Here's how the part is built. I have some questions about the finished solid (model axes, mm). A direction names the side the tool comes from. Coordinates: 2 decimals unless noted, no trailing zeros. Order: outer loops, then holes, each group sorted by start corner. A loop starts at its lowest first (then second) coordinate and runs counter-clockwise, first axis right, second up. Notation, with made-up numbers: M 83.5,-19 L 100.5,-19 A12 ccw 100.5,-14 Z; hole C 77,-19.5 d3. An arc over 180 degrees is marked long. One line per question, with ' | ' between items. Start each with the question number.
```python
from build123d import *

# Parameters (mm, degrees)
BOSS_EXTRUDE1_DEPTH = 3


with BuildPart() as part:
    # Sketch1 → Boss-Extrude1 (new body)
    with BuildSketch(Plane(origin=(0, 0, 0), x_dir=(1, 0, 0), z_dir=(0, 1, 0))):
        with BuildLine():
            Line((-27.566533023, 9.36), (-27.566533023, 0))
            Line((-27.566533023, 0), (-19.823403694, 0))
            ThreePointArc((-19.823403694, 0), (24.20597109, 6.306968985), (65.433466977, 23))
            ThreePointArc((65.433466977, 23), (73.082886665, 22.390495512), (80.646880945, 23.683208869))
            ThreePointArc((80.646880945, 23.683208869), (81.946672363, 24.893615616), (81.784737476, 26.662321164))
            ThreePointArc((81.784737476, 26.662321164), (78.82438559, 31.885442154), (76.202135766, 37.28622747))
            ThreePointArc((76.202135766, 37.28622747), (86.37958616, 41.621825), (95.668579031, 47.629529544))
            ThreePointArc((95.668579031, 47.629529544), (96.113926531, 48.706505439), (95.666017221, 49.782418412))
            ThreePointArc((95.666017221, 49.782418412), (89.924608564, 54.937742393), (85.709789242, 61.401211803))
            ThreePointArc((85.709789242, 61.401211803), (96.000732533, 71.797200989), (102.357305132, 84.971952969))
            ThreePointArc((102.357305132, 84.971952969), (102.11128314, 86.223857216), (101.047487459, 86.928222044))
            ThreePointArc((101.047487459, 86.928222044), (95.950995205, 87.647987285), (90.808707622, 87.869738741))
            ThreePointArc((90.808707622, 87.869738741), (100.106213422, 97.05037675), (104.313081391, 109.420905852))
            ThreePointArc((104.313081391, 109.420905852), (104.396564886, 110.399625231), (103.439203659, 110.619444698))
            ThreePointArc((103.439203659, 110.619444698), (98.285170112, 109.227963636), (93.040390076, 110.224238556))
            ThreePointArc((93.040390076, 110.224238556), (96.824995658, 122.538102913), (96.530215503, 135.417062479))
            ThreePointArc((96.530215503, 135.417062479), (95.551508519, 136.778926007), (93.878347384, 136.893256429))
            ThreePointArc((93.878347384, 136.893256429), (83.613278323, 129.68205398), (77.858466896, 118.535071023))
            ThreePointArc((77.858466896, 118.535071023), (74.985694546, 124.095226744), (72.596248771, 129.879576449))
            ThreePointArc((72.596248771, 129.879576449), (70.378357546, 131.020039942), (68.639848531, 129.231944623))
            ThreePointArc((68.639848531, 129.231944623), (67.651272843, 114.747827583), (68.577278714, 100.25957574))
            ThreePointArc((68.577278714, 100.25957574), (63.407288288, 102.259220756), (59.026108144, 105.655195101))
            ThreePointArc((59.026108144, 105.655195101), (56.300849607, 106.738729111), (54.315586254, 104.580069929))
            ThreePointArc((54.315586254, 104.580069929), (55.34526323, 85.900059583), (63.427341461, 69.02750694))
            Line((63.427341461, 69.02750694), (44.822180162, 73.063888147))
            ThreePointArc((44.822180162, 73.063888147), (43.189327409, 72.023710618), (42.770208924, 70.133600278))
            Line((42.770208924, 70.133600278), (51.693414268, 52.061516653))
            ThreePointArc((51.693414268, 52.061516653), (51.807398335, 49.244580753), (49.792960169, 47.272232126))
            ThreePointArc((49.792960169, 47.272232126), (43.886083409, 53.379891607), (36.716738418, 57.940065925))
            ThreePointArc((36.716738418, 57.940065925), (34.842559279, 58.150522241), (35.17981611, 56.294963797))
            ThreePointArc((35.17981611, 56.294963797), (38.195000716, 47.026649531), (37.963262453, 37.282970301))
            ThreePointArc((37.963262453, 37.282970301), (36.915972263, 35.842205611), (35.471592941, 36.884504997))
            ThreePointArc((35.471592941, 36.884504997), (32.374331301, 43.249850807), (27.655103234, 48.526169922))
            ThreePointArc((27.655103234, 48.526169922), (26.369610718, 48.570167749), (26.028819046, 47.329890419))
            ThreePointArc((26.028819046, 47.329890419), (26.962894841, 38.326203111), (22.69935772, 30.341146196))
            ThreePointArc((22.69935772, 30.341146196), (21.519458622, 30.046407872), (20.701006485, 30.9459459))
            ThreePointArc((20.701006485, 30.9459459), (18.760748853, 37.885894085), (15.830732782, 44.469395153))
            ThreePointArc((15.830732782, 44.469395153), (14.897444009, 44.903650637), (14.219241967, 44.129281378))
            ThreePointArc((14.219241967, 44.129281378), (11.765539078, 35.905199886), (6.117654668, 29.443189676))
            ThreePointArc((6.117654668, 29.443189676), (4.728143423, 29.340639166), (4.041804517, 30.553155976))
            ThreePointArc((4.041804517, 30.553155976), (3.570156048, 36.827406443), (1.56510947, 42.791336307))
            ThreePointArc((1.56510947, 42.791336307), (0.867859685, 43.215318025), (0.196498979, 42.751429503))
            ThreePointArc((0.196498979, 42.751429503), (-10.860043289, 29.237113049), (-27.566533023, 24.16))
            Line((-27.566533023, 24.16), (-27.566533023, 12.36))
            Line((-27.566533023, 12.36), (-16.746533023, 12.36))
            ThreePointArc((-16.746533023, 12.36), (-15.246533023, 10.86), (-16.746533023, 9.36))
            Line((-16.746533023, 9.36), (-27.566533023, 9.36))
        make_face()
    extrude(amount=BOSS_EXTRUDE1_DEPTH)


solid = part.part
```
1. We'd pull the mould along X, two halves only. Please class faces 1 (the face through (-27.567, 1, -5)), 2 (the face through (95.88, 1.48, -71.63)), 3 (the face through (38.175, 1.479, -47.162)), 4 (the face through (47.17, 1.48, -61.22)): released by +X, released by -X, zero draft, split by the parting line, or undercut.
2. Will these pins go through, and if not, where does the flat tip stop? pin 1 (0.9 mm diameter, centred on x = -25, y = 2, fed in from -Z); pin 2 (1 mm diameter, centred on x = 77.5, y = 2, fed in from -Z).
3. Which directions (+Z, -Z, +X, -X, +Y, -Y) give clear straight access to the entire face, cutting with the end or side of a thin tool? Please do faces 5 (the face through (43.978, 1.479, -53.304)), 6 (the face through (89.995, 1.479, -54.856)), 7 (the face through (-22, 1, -9.36)), 8 (the face through (72.975, 1.479, -22.386)).
4. Imagine slicing it at B-B (z = -16.5). List the corners of the cut face in (x, y) for me, then the cut area to 3 significant figures.
5. I need wall thicknesses on line 1 (X direction, y = 2.7, z = -44); line 2 (Z direction, x = 76.5, y = 0.8); line 3 (X direction, y = 2.1, z = -46). Which ranges of each line are inside material? Lowest first, please.
6. Imagine slicing it at A-A (z = -124.5). List the corners of the cut face in (x, y) for me, then the cut area to 3 significant figures.
Entries:
1) face 1: released by -X | face 2: released by +X | face 3: undercut | face 4: undercut
2) pin 1: z = -24.31 | pin 2: z = -120.08
3) face 5: +Y, -Y | face 6: +X, +Y, -Y | face 7: -X, +Y, -Y | face 8: +Z, +Y, -Y
4) outline: M -27.57,0 L 52.53,0 L 52.53,3 L -27.57,3 Z | area: 240 mm²
5) line 1: 14.21 to 16.08, 27.01 to 31.85, 38.48 to 90.48 | line 2: -121.02 to -37.38, -36.63 to -22.73 | line 3: 26.52 to 30.24, 38.33 to 93.47
6) outline: M 68.11,0 L 74.8,0 L 74.8,3 L 68.11,3 Z; M 80.08,0 L 97.05,0 L 97.05,3 L 80.08,3 Z | area: 71.0 mm²
